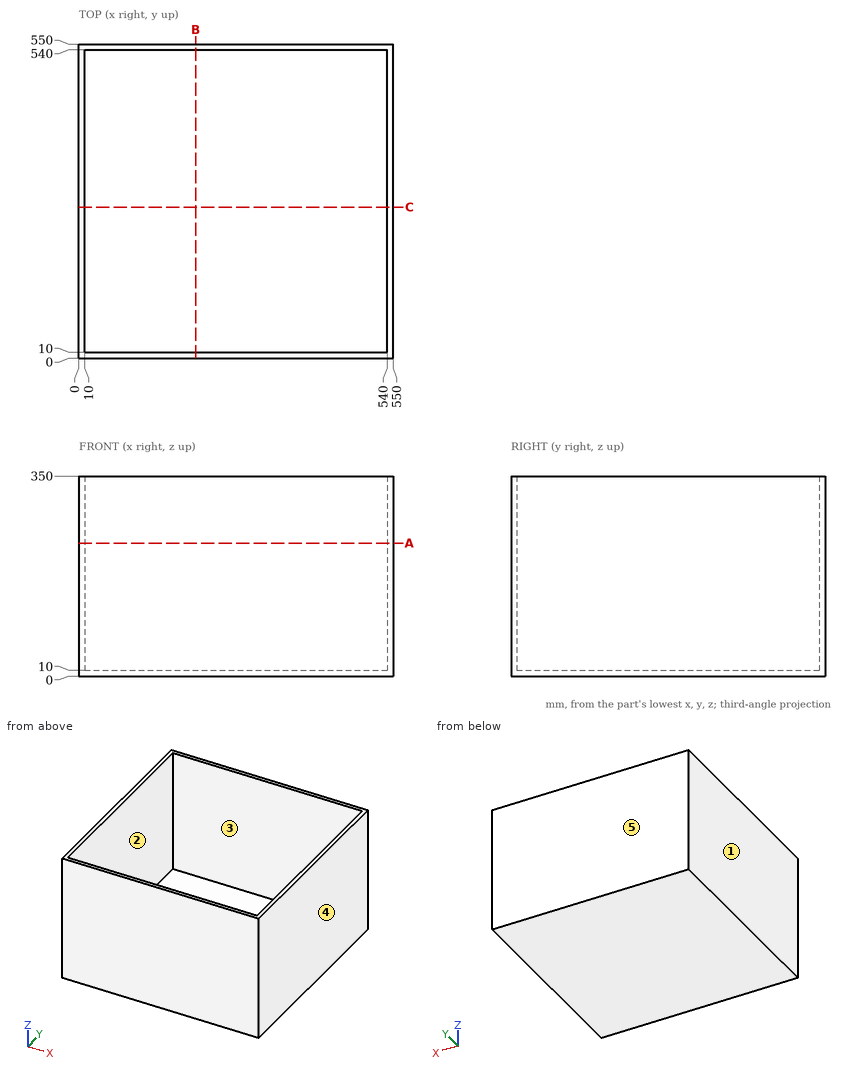
Part print with two shaded views. Sizes in mm from the minimum x, y, z corner. A direction names the side the tool comes from. Give positions to 0.01 mm unless a question says otherwise; leave off trailing zeros. Order: outer loops, then holes, each group sorted by start corner. A loop starts at its lowest first (then second) coordinate and runs counter-clockwise, first axis right, second up. Notation, with made-up numbers: M 53.5,-32.75 L 110.5,-32.75 A33 ccw 110.5,1.25 Z; hole C 19.5,-22.5 d2. An arc over 180 degrees is marked long. Put each result on its own line as item: value.
Item 1: Which spindle directions (+Z, -Z, +X, -X, +Y, -Y) get a long thin tool onto all of the face, cutting with end or side? Do the marked faces 1 and 2. Say none if no direction does.
Results are:
face 1: +Z, -Z, -X, +Y, -Y
face 2: +Z
Item 2: Cut at A-A on z = 232.5. Write the cut outline in (x, y), then the cut area to 3 significant figures.
Results are:
outline: M 0,0 L 550,0 L 550,550 L 0,550 Z; hole M 10,10 L 540,10 L 540,540 L 10,540 Z
area: 21,600 mm2
Item 3: Wall check: probe 1 along Y at (x, z) = (314, 69.5); probe 2 along Z at (x, y) = (186, 200). Give the ranges that are in metal, low to high.
Results are:
probe 1: 0 to 10, 540 to 550
probe 2: 0 to 10
Item 4: Drop a flat-ended pin along its axis: pin 1 Ø12 at (x, y) = (471.5, 58.5) entering from -Z. Give the stop position or say it passes through.
Results are:
pin 1: z = 0
Item 5: Cut at B-B on x = 204.5. Write the cut outline in (y, z).
Results are:
outline: M 0,0 L 550,0 L 550,350 L 540,350 L 540,10 L 10,10 L 10,350 L 0,350 Z
Item 6: Pull direction X, two halves, no side cores. Call the marked faces 3, 4 and 5: +X half, -X half, draft (parallel to the pull), parting line (faces both ways), or undercut.
Results are:
face 3: undercut
face 4: +X half
face 5: draft
